Here's the drawing with two shaded views (mm, measured from the low corner). I have some questions. Give positions to 0.01 mm unless a question says otherwise; leave off trailing zeros. Write each loop counter-clockwise with the first axis right and the second up, starting at its lowest first coordinate (ties: lowest second). Pieces come first, ordered by that corner, then holes.
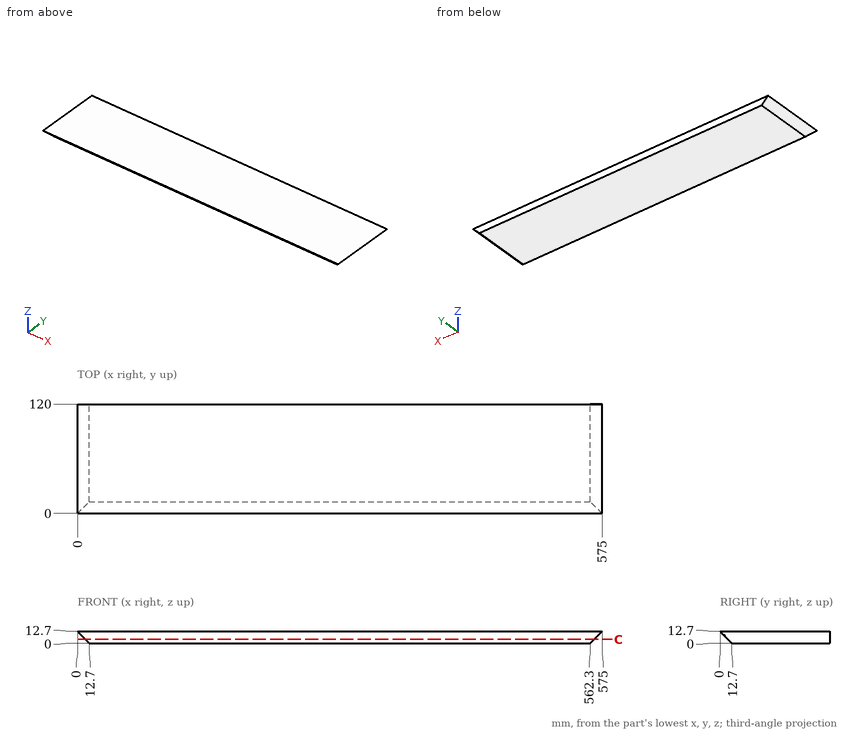
1) Suppose I cut it at C-C on z = 4. Write out the boundary of the cut face in (x, y), plus the area to 3 significant figures.
Values follow:
outline: (8.7, 8.7) - (566.3, 8.7) - (566.3, 120) - (8.7, 120) - close
area: 62,100 mm2
2) Please list where these lines run through material, in increasing order: L1, parallel to X at y = 73.5, z = 3; L2, parallel to X at y = 37, z = 9.5; L3, parallel to Y at x = 543.5, z = 4.5.
Values follow:
L1: x = 9.7 to 565.3
L2: x = 3.2 to 571.8
L3: y = 8.2 to 120
3) For pin 1 Ø6 at (y, z) = (101, 2.5) entering from -X; pin 2 Ø5 at (x, z) = (352, 6) entering from -Y; pin 3 Ø3 at (y, z) = (61.5, 2.5) entering from +X; pin 4 Ø6 at (y, z) = (24.5, 10) entering from +X, each with a flat end and sliding along its axis, tell me the tip position at first contact or that it passes through.
Values follow:
pin 1: stops at x = 7.2
pin 2: stops at y = 4.2
pin 3: stops at x = 566.3
pin 4: stops at x = 575
